```python
from build123d import *

# Parameters (mm, degrees)
SKETCH1_W               = 124.63
SKETCH1_H               = 304.8
BASE_FLANGE1_DEPTH      = 1.57
EDGE_FLANGE1_DEPTH      = 304.8
EDGE_FLANGE1_BEND_DEPTH = 304.8
FILLET1_R               = 6.35
HOLE1_START             = -64.645
HOLE1_OUTLINE_R         = 1.5
HOLE1_DEPTH             = 129.29
HOLE2_START             = -64.645
HOLE2_OUTLINE_R         = 1.5
HOLE2_DEPTH             = 129.29
SKETCH18_R              = 1.5
CUT_EXTRUDE1_DEPTH      = 10
SKETCH19_R              = 1.5
CUT_EXTRUDE2_DEPTH      = 10


# Read off the part's stored shape, not the designer's step: Hole1, Hole2
# Sheet-metal steps are written as plain solids
with BuildPart() as part:
    # Sketch1 → Base-Flange1 (new body)
    with BuildSketch(Plane(origin=(0, 0, 0), x_dir=(0, 0, -1), z_dir=(1, 0, 0))):
        Rectangle(SKETCH1_W, SKETCH1_H)
    extrude(amount=BASE_FLANGE1_DEPTH)

    # Edge-Flange1 section (across the edge) → Edge-Flange1 (add)
    with BuildSketch(Plane(origin=(0, -152.4, 63.075), x_dir=(0, 0, -1), z_dir=(0, 1, 0))):
        with BuildLine():
            Line((-1.57, 0.76), (-1.57, 59.18))
            Line((-1.57, 59.18), (0, 59.18))
            Line((0, 59.18), (0, 0.76))
            ThreePointArc((0, 0.76), (0.222598846, 0.222598846), (0.76, 0))
            Line((0.76, 0), (0.76, -1.57))
            ThreePointArc((0.76, -1.57), (-0.8875588, -0.8875588), (-1.57, 0.76))
        make_face()
    extrude(amount=EDGE_FLANGE1_DEPTH)

    # Edge-Flange1 section 2 (across the edge) → Edge-Flange1 bend (add)
    with BuildSketch(Plane(origin=(0, 152.4, -63.075), x_dir=(0, 0, 1), z_dir=(0, -1, 0))):
        with BuildLine():
            Line((-1.57, 0.76), (-1.57, 59.18))
            Line((-1.57, 59.18), (0, 59.18))
            Line((0, 59.18), (0, 0.76))
            ThreePointArc((0, 0.76), (0.222598846, 0.222598846), (0.76, 0))
            Line((0.76, 0), (0.76, -1.57))
            ThreePointArc((0.76, -1.57), (-0.8875588, -0.8875588), (-1.57, 0.76))
        make_face()
    extrude(amount=EDGE_FLANGE1_BEND_DEPTH)

    # Fillet1
    fillet1_edges = [part.edges().sort_by_distance(p)[0] for p in [
        (-59.18, -152.4, 63.86),
        (-59.18, -152.4, -63.86),
    ]]
    fillet(fillet1_edges, radius=FILLET1_R)

    # Hole1 outline → Hole1 (cut)
    with BuildSketch(Plane.XY.offset(HOLE1_START)):
        with Locations((-8.39, -146.37)):
            Circle(HOLE1_OUTLINE_R)
        with Locations((-41.86, -146.37)):
            Circle(HOLE1_OUTLINE_R)
    extrude(amount=HOLE1_DEPTH, mode=Mode.SUBTRACT)

    # Hole2 outline → Hole2 (cut)
    with BuildSketch(Plane.XY.offset(HOLE2_START)):
        with Locations((-53.95, 147.08)):
            Circle(HOLE2_OUTLINE_R)
        with Locations((-8.38, 147.08)):
            Circle(HOLE2_OUTLINE_R)
        with Locations((-8.38, 99.28)):
            Circle(HOLE2_OUTLINE_R)
        with Locations((-53.95, 99.28)):
            Circle(HOLE2_OUTLINE_R)
    extrude(amount=HOLE2_DEPTH, mode=Mode.SUBTRACT)

    # Sketch18 → Cut-Extrude1 (cut)
    with BuildSketch(Plane(origin=(1.57, 0, 0), x_dir=(0, 0, -1), z_dir=(1, 0, 0))):
        with Locations((52.085, -146.37)):
            Circle(SKETCH18_R)
    cut_extrude1 = extrude(amount=-CUT_EXTRUDE1_DEPTH, mode=Mode.SUBTRACT)

    # Mirror1: Cut-Extrude1 across plane
    add(cut_extrude1.mirror(Plane.XY), mode=Mode.SUBTRACT)

    # Sketch19 → Cut-Extrude2 (cut)
    with BuildSketch(Plane(origin=(1.57, 0, 0), x_dir=(0, 0, -1), z_dir=(1, 0, 0))):
        with Locations((52.085, 99.28)):
            Circle(SKETCH19_R)
        with Locations((-52.085, 99.28)):
            Circle(SKETCH19_R)
    extrude(amount=-CUT_EXTRUDE2_DEPTH, mode=Mode.SUBTRACT)


solid = part.part
```
Check sheet for the modelled part. Datum: model origin and axes. Units: mm. A direction names the side the tool comes from. Coordinates: 2 decimals unless noted, no trailing zeros. Write each loop counter-clockwise with the first axis right and the second up, starting at its lowest first coordinate (ties: lowest second). Pieces come first, ordered by that corner, then holes. Notation, with made-up numbers: (15.5, -34) -> (36.5, -34) arc R29 cw to (36.5, -11) -> close; hole circle Ø2 at (28.25, 86). An arc over 180 degrees is marked (long way). Use a Markdown table: item, result.
1. Scan lines: line 1 along Y through (x, z) = (-8.38, 63.55); line 2 along Z through (x, y) = (-37, 43.5) (3 decimals); line 3 along Y through (x, z) = (-41.86, 63.6). Record each from-to range of solid material in increasing order.
Reported:
| item | result |
|---|---|
| line 1 | y = -152.4 to -147.87, -144.87 to 97.78, 100.78 to 145.58, 148.58 to 152.4 |
| line 2 | z = -64.645 to -63.075, 63.075 to 64.645 |
| line 3 | y = -152.4 to -147.87, -144.87 to 152.4 |
2. Sectioned sample at A-A (y = 69). Enter the section's corners in (x, z) (3 decimals).
Reported:
| item | result |
|---|---|
| outline | (-59.18, -64.645) -> (-0.76, -64.645) arc R2.33 ccw to (1.57, -62.315) -> (1.57, 62.315) arc R2.33 ccw to (-0.76, 64.645) -> (-59.18, 64.645) -> (-59.18, 63.075) -> (-0.76, 63.075) arc R0.76 cw to (0, 62.315) -> (0, -62.315) arc R0.76 cw to (-0.76, -63.075) -> (-59.18, -63.075) -> close |
3. Release check for a two-part mould opening along Z. For faces 3 (the flat face through (-30, -2, 63.075)), 4 (the flat face through (-30, -2, 64.645)), 5 (the cylindrical face through (-57.37, -150.49, -63.85)) record: pulls with the +Z half, pulls with the -Z half, needs draft (parallel to the pull), parting line crosses it, or undercut.
Reported:
| item | result |
|---|---|
| face 3 | undercut |
| face 4 | pulls with the +Z half |
| face 5 | needs draft |
4. Sectioned sample at B-B (z = -2). Enter the section's corners in (x, y), plus the area to 3 significant figures.
Reported:
| item | result |
|---|---|
| outline | (0, -152.4) -> (1.57, -152.4) -> (1.57, 152.4) -> (0, 152.4) -> close |
| area | 479 mm2 |
5. Go/stop test with flat-tipped pins: pin 1 Ø1 at (y, z) = (-19.5, -30.5) entering from -X; pin 2 Ø2.5 at (y, z) = (99.28, 52.085) entering from +X. Record where each tip stops, or that it passes through.
Reported:
| item | result |
|---|---|
| pin 1 | stops at x = 0 |
| pin 2 | passes through |
6. Tool access check on faces 1 (the flat face through (-30, 2, -63.075)), 2 (the flat face through (1.57, 2, 1)). Record the directions out of +Z, -Z, +X, -X, +Y, -Y that give a thin tool (end or side, any length) a straight path to the whole face; none if there is none.
Reported:
| item | result |
|---|---|
| face 1 | -X, +Y, -Y |
| face 2 | +Z, -Z, +X, +Y, -Y |
